Part model, mm, in its own coordinate system. A direction names the side the tool comes from. Round coordinates to 2 decimals unless told otherwise and drop trailing zeros. Write each loop counter-clockwise with the first axis right and the second up, starting at its lowest first coordinate (ties: lowest second). Pieces come first, ordered by that corner, then holes.
1) Saw through at B-B on z = 0. Write the cut outline in (x, y), and give its area (3 significant figures).
2) Saw through at A-A on y = 0. Write the cut outline in (x, z), and give its area (3 significant figures).
3) Saw through at C-C on x = 1.7. Write the cut outline in (y, z), and give its area (3 significant figures).
4) Drill centre lines: L1, parallel to Z at x = 1.3, y = -9; L2, parallel to Z at x = 1, y = -7.25; L3, parallel to Y at x = 1.5, z = 7.5. Where is each one in solid material? Low to high.
5) Saw through at D-D on z = 12. Write the cut outline in (x, y), and give its area (3 significant figures).
6) Which spindle directions (+Z, -Z, +X, -X, +Y, -Y) get a long thin tool onto all of the face, cutting with end or side? Do faces 5 (the flat face through (1, 3, 17.35)), 6 (the flat face through (2, -8, 0)). Say none if no direction does.
7) Pull direction Y, two halves, no side cores. Call faces 1 (the flat face through (1, -2.933, 0)), 2 (the flat face through (0, -8, 0)), 3 (the cylindrical face through (0.99, -9.95, 8.81)), 4 (the cylindrical face through (0.99, -19.99, 0.59)): +Y half, -Y half, draft (parallel to the pull), parting line (faces both ways), or undercut.
```python
from build123d import *

# Parameters (mm, degrees)
SKETCH1_R           = 20
SKETCH1_R_2         = 1.5
BOSS_EXTRUDE1_DEPTH = 2
SKETCH3_W           = 34.7
SKETCH3_H           = 20.283452378
CUT_EXTRUDE1_DEPTH  = 29.354893758


with BuildPart() as part:
    # Sketch1 → Boss-Extrude1 (new body)
    with BuildSketch(Plane(origin=(0, 0, 0), x_dir=(0, 0, -1), z_dir=(1, 0, 0))):
        Circle(SKETCH1_R)
        with Locations((0, 14.75)):
            Circle(SKETCH1_R_2, mode=Mode.SUBTRACT)
        with Locations((14.75, 0)):
            Circle(SKETCH1_R_2, mode=Mode.SUBTRACT)
        with Locations((0, -14.75)):
            Circle(SKETCH1_R_2, mode=Mode.SUBTRACT)
        with Locations((-14.75, 0)):
            Circle(SKETCH1_R_2, mode=Mode.SUBTRACT)
        with Locations((-8.485281374, 8.485281374)):
            Circle(SKETCH1_R_2, mode=Mode.SUBTRACT)
        with Locations((8.485281374, 8.485281374)):
            Circle(SKETCH1_R_2, mode=Mode.SUBTRACT)
        with Locations((8.485281374, -8.485281374)):
            Circle(SKETCH1_R_2, mode=Mode.SUBTRACT)
        with Locations((-8.485281374, -8.485281374)):
            Circle(SKETCH1_R_2, mode=Mode.SUBTRACT)
    extrude(amount=BOSS_EXTRUDE1_DEPTH)

    # Sketch3 → Cut-Extrude1 (cut, through all)
    with BuildSketch(Plane(origin=(2, 0, 0), x_dir=(0, 0, -1), z_dir=(1, 0, 0))):
        with Locations((0, 7.208273811)):
            Rectangle(SKETCH3_W, SKETCH3_H)
    extrude(amount=-CUT_EXTRUDE1_DEPTH, mode=Mode.SUBTRACT)


with BuildPart() as cut_extrude1_kept_piece:
    # of the separate pieces the step leaves, the one the design keeps (cut_extrude1_pieces_kept)
    add(part.part.solids().sort_by_distance((0, 9.948743639, 17.35))[0])


solid = cut_extrude1_kept_piece.part
```
Completed:
1. outline: (0, -20) - (2, -20) - (2, -16.25) - (0, -16.25) - close; (0, -13.25) - (2, -13.25) - (2, -2.93) - (0, -2.93) - close
1. area: 28.1 mm2
2. outline: (0, -20) - (2, -20) - (2, -17.35) - (0, -17.35) - close; (0, 17.35) - (2, 17.35) - (2, 20) - (0, 20) - close
2. area: 10.6 mm2
3. outline: (-2.93, -17.35) - (-2.93, 17.35) - (9.95, 17.35) arc R20 ccw (long way) to (9.95, -17.35) - close; hole circle Ø3 at (-14.75, 0); hole circle Ø3 at (-8.49, -8.49); hole circle Ø3 at (-8.49, 8.49)
3. area: 541 mm2
4. L1: z = -17.86 to -9.89, -7.08 to 7.08, 9.89 to 17.86
4. L2: z = -18.64 to -9.34, -7.63 to 7.63, 9.34 to 18.64
4. L3: y = -18.54 to -9.62, -7.35 to -2.93
5. outline: (0, -16) - (2, -16) - (2, -2.93) - (0, -2.93) - close
5. area: 26.1 mm2
6. face 5: +X, -X, +Y
6. face 6: +Z, -Z, +X, +Y, -Y
7. face 1: +Y half
7. face 2: draft
7. face 3: undercut
7. face 4: parting line
